Check sheet for the modelled part. Datum: model origin and axes. Units: mm. Round coordinates to 2 decimals unless told otherwise and drop trailing zeros. Loops run counter-clockwise (first coordinate to the right, second up) from the corner with the lowest first, then second, coordinate; pieces in that order, holes last. Notation, with made-up numbers: (-5, 80.5) - (21, 80.5) arc R14 cw to (21, 89.5) - close; hole circle Ø2 at (-21, -6). An arc over 180 degrees is marked (long way). Return JSON: item names as keys, results as strings.
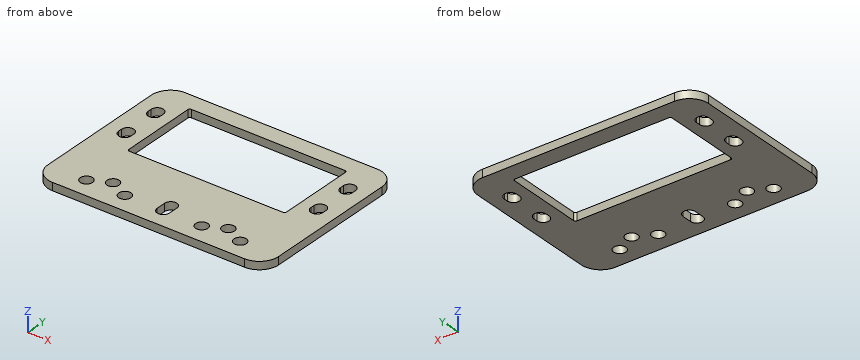
from build123d import *

# Parameters (mm, degrees)
SKETCH1_W           = 60
SKETCH1_H           = 45
BOSS_EXTRUDE1_DEPTH = 2.032
FILLET1_R           = 5
SKETCH2_W           = 41
SKETCH2_H           = 21
CUT_EXTRUDE1_DEPTH  = 3.032
FILLET2_R           = 0.5
CUT_EXTRUDE2_DEPTH  = 3.032
SKETCH4_R           = 1.6
CUT_EXTRUDE3_DEPTH  = 3.032


with BuildPart() as part:
    # Sketch1 → Boss-Extrude1 (new body)
    with BuildSketch(Plane.XY):
        Rectangle(SKETCH1_W, SKETCH1_H)
    extrude(amount=BOSS_EXTRUDE1_DEPTH)

    # Fillet1
    fillet1_edges = [part.edges().sort_by_distance(p)[0] for p in [
        (30, -22.5, 1.016),
        (-30, -22.5, 1.016),
        (-30, 22.5, 1.016),
        (30, 22.5, 1.016),
    ]]
    fillet(fillet1_edges, radius=FILLET1_R)

    # Sketch2 → Cut-Extrude1 (cut, through all)
    with BuildSketch(Plane.XY.offset(2.032)):
        with Locations((0, 7.5)):
            Rectangle(SKETCH2_W, SKETCH2_H)
    extrude(amount=-CUT_EXTRUDE1_DEPTH, mode=Mode.SUBTRACT)

    # Fillet2
    fillet2_edges = [part.edges().sort_by_distance(p)[0] for p in [
        (20.5, 18, 1.016),
        (20.5, -3, 1.016),
        (-20.5, -3, 1.016),
        (-20.5, 18, 1.016),
    ]]
    fillet(fillet2_edges, radius=FILLET2_R)

    # Sketch3 → Cut-Extrude2 (cut, through all)
    with BuildSketch(Plane.XY.offset(2.032)):
        with BuildLine():
            Line((-23.4, 3), (-23.4, 2))
            ThreePointArc((-23.4, 2), (-25, 0.4), (-26.6, 2))
            Line((-26.6, 2), (-26.6, 3))
            ThreePointArc((-26.6, 3), (-25, 4.6), (-23.4, 3))
        make_face()
        with BuildLine():
            Line((-23.4, 12), (-23.4, 13))
            ThreePointArc((-23.4, 13), (-25, 14.6), (-26.6, 13))
            Line((-26.6, 13), (-26.6, 12))
            ThreePointArc((-26.6, 12), (-25, 10.4), (-23.4, 12))
        make_face()
        with BuildLine():
            Line((23.4, 3), (23.4, 2))
            ThreePointArc((23.4, 2), (25, 0.4), (26.6, 2))
            Line((26.6, 2), (26.6, 3))
            ThreePointArc((26.6, 3), (25, 4.6), (23.4, 3))
        make_face()
        with BuildLine():
            Line((23.4, 12), (23.4, 13))
            ThreePointArc((23.4, 13), (25, 14.6), (26.6, 13))
            Line((26.6, 13), (26.6, 12))
            ThreePointArc((26.6, 12), (25, 10.4), (23.4, 12))
        make_face()
    extrude(amount=-CUT_EXTRUDE2_DEPTH, mode=Mode.SUBTRACT)

    # Sketch4 → Cut-Extrude3 (cut, through all)
    with BuildSketch(Plane.XY.offset(2.032)):
        with Locations((-15, -15)):
            Circle(SKETCH4_R)
        with Locations((15, -15)):
            Circle(SKETCH4_R)
        with Locations((10, -17.5)):
            Circle(SKETCH4_R)
        with Locations((-10, -17.5)):
            Circle(SKETCH4_R)
        with Locations((20, -17.5)):
            Circle(SKETCH4_R)
        with Locations((-20, -17.5)):
            Circle(SKETCH4_R)
        with BuildLine():
            Line((1.6, -15), (1.6, -17.5))
            ThreePointArc((1.6, -17.5), (0, -19.1), (-1.6, -17.5))
            Line((-1.6, -17.5), (-1.6, -15))
            ThreePointArc((-1.6, -15), (0, -13.4), (1.6, -15))
        make_face()
    extrude(amount=-CUT_EXTRUDE3_DEPTH, mode=Mode.SUBTRACT)


solid = part.part
Q1. Sectioned sample at A-A (x = -10). Enter the section's corners in (y, z), plus the area to 3 significant figures.
Answer key:
{"outline": "(-22.5, 0) - (-19.1, 0) - (-19.1, 2.03) - (-22.5, 2.03) - close; (-15.9, 0) - (-3, 0) - (-3, 2.03) - (-15.9, 2.03) - close; (18, 0) - (22.5, 0) - (22.5, 2.03) - (18, 2.03) - close", "area": "42.3 mm²"}
Q2. Scan lines: probe 1 along Y at (x, z) = (-10, 1); probe 2 along Y at (x, z) = (15, 1); probe 3 along Y at (x, z) = (2.5, 1.45). Record each from-to range of solid material in increasing order. Write a range as [from, to].
Answer key:
{"probe 1": "y = [-22.5, -19.1], [-15.9, -3], [18, 22.5]", "probe 2": "y = [-22.5, -16.6], [-13.4, -3], [18, 22.5]", "probe 3": "y = [-22.5, -3], [18, 22.5]"}
Q3. Depth check by flat-ended pin: P1, Ø8, axis at x = 16, y = 13, coming from the +Z side. Enter the tip coordinate at first touch or a pass-through.
Answer key:
{"P1": "passes through"}
Q4. Sectioned sample at B-B (z = 1.3). State how many separate pieces and enclosed holes the cut face has, plus the area to 3 significant figures.
Answer key:
{"separate pieces": "1", "enclosed holes": "12", "area": "1,710 mm²"}
